from build123d import *

# Parameters (mm, degrees)
SKETCH_2_R           = 3
SKETCH_2_R_2         = 2.5
SKETCH_2_R_3         = 2.55
SKETCH_2_W           = 6
SKETCH_2_H           = 6
SKETCH_2_W_2         = 6.1
SKETCH_2_H_2         = 2
EXTRUDE_2_DEPTH      = 8.5
CHAMFER_3_SIZE       = 2.5
FILLET_1_R           = 3
CUT_EXTRUDE_1_DEPTH  = 1.2
SKETCH_4_R           = 0.85
CUT_EXTRUDE_2_DEPTH  = 5
CUT_EXTRUDE_3_DEPTH  = 1.2
SKETCH_6_R           = 0.85
CUT_EXTRUDE_4_DEPTH  = 5
FILLET_2_R           = 2
SKETCH_7_W           = 6.1
SKETCH_7_H           = 10
CUT_EXTRUDE_5_DEPTH  = 2
SKETCH_8_R           = 0.85
CUT_EXTRUDE_6_DEPTH  = 5
SKETCH_9_R           = 3.65
CUT_EXTRUDE_7_DEPTH  = 2.5
SKETCH_10_R          = 3.65
CUT_EXTRUDE_8_DEPTH  = 2.5
SKETCH_11_R          = 5
CUT_EXTRUDE_9_DEPTH  = 2.5
SKETCH_12_R          = 5
CUT_EXTRUDE_10_DEPTH = 2.5
CHAMFER_4_SIZE       = 0.5
CHAMFER_5_SIZE       = 0.3


with BuildPart() as part:
    # 草图2 → 凸台-拉伸2 (new body)
    with BuildSketch(Plane.XY):
        with BuildLine():
            Line((-10.9, 9.1), (25.9, 9.1))
            ThreePointArc((25.9, 9.1), (29.435533906, 10.564466094), (30.9, 14.1))
            Line((30.9, 14.1), (30.9, 29.1))
            ThreePointArc((30.9, 29.1), (32.364466094, 32.635533906), (35.9, 34.1))
            Line((35.9, 34.1), (44.1, 34.1))
            ThreePointArc((44.1, 34.1), (47.635533906, 32.635533906), (49.1, 29.1))
            Line((49.1, 29.1), (49.1, 9.1))
            Line((49.1, 9.1), (49.1, -45.9))
            ThreePointArc((49.1, -45.9), (47.635533906, -49.435533906), (44.1, -50.9))
            Line((44.1, -50.9), (-4.1, -50.9))
            ThreePointArc((-4.1, -50.9), (-7.635533906, -49.435533906), (-9.1, -45.9))
            Line((-9.1, -45.9), (-9.1, -14.1))
            ThreePointArc((-9.1, -14.1), (-10.564466094, -10.564466094), (-14.1, -9.1))
            Line((-14.1, -9.1), (-30.9, -9.1))
            ThreePointArc((-30.9, -9.1), (-34.435533906, -7.635533906), (-35.9, -4.1))
            Line((-35.9, -4.1), (-35.9, 4.1))
            ThreePointArc((-35.9, 4.1), (-34.435533906, 7.635533906), (-30.9, 9.1))
            Line((-30.9, 9.1), (-10.9, 9.1))
        make_face()
        Circle(SKETCH_2_R, mode=Mode.SUBTRACT)
        with Locations((40, 0)):
            Circle(SKETCH_2_R_2, mode=Mode.SUBTRACT)
        with Locations((0, -40)):
            Circle(SKETCH_2_R, mode=Mode.SUBTRACT)
        with Locations((40, -40)):
            Circle(SKETCH_2_R_3, mode=Mode.SUBTRACT)
        with Locations((40, 25)):
            Circle(SKETCH_2_R_3, mode=Mode.SUBTRACT)
        with Locations((-26.8, 0)):
            Circle(SKETCH_2_R_3, mode=Mode.SUBTRACT)
        with Locations((20, -20)):
            Rectangle(SKETCH_2_W, SKETCH_2_H, mode=Mode.SUBTRACT)
        with Locations((20, -40.9)):
            Rectangle(SKETCH_2_W_2, SKETCH_2_H_2, mode=Mode.SUBTRACT)
    extrude(amount=EXTRUDE_2_DEPTH)

    # 倒角3
    chamfer_3_edges = [part.edges().sort_by_distance(p)[0] for p in [
        (37.5, 0, 0),
        (37.45, -40, 8.5),
        (37.45, 25, 8.5),
        (-29.35, 0, 0),
    ]]
    chamfer(chamfer_3_edges, length=CHAMFER_3_SIZE)

    # 圆角1
    fillet_1_edges = [part.edges().sort_by_distance(p)[0] for p in [
        (20, -41.9, 0),
    ]]
    fillet(fillet_1_edges, radius=FILLET_1_R)

    # 草图3 → 切除-拉伸1 (cut)
    with BuildSketch(Plane.XY.offset(8.5)):
        with BuildLine():
            Line((15.9, -11.9), (24.1, -11.9))
            ThreePointArc((24.1, -11.9), (24.807106781, -12.192893219), (25.1, -12.9))
            Line((25.1, -12.9), (25.1, -27.1))
            ThreePointArc((25.1, -27.1), (24.807106781, -27.807106781), (24.1, -28.1))
            Line((24.1, -28.1), (15.9, -28.1))
            ThreePointArc((15.9, -28.1), (15.192893219, -27.807106781), (14.9, -27.1))
            Line((14.9, -27.1), (14.9, -12.9))
            ThreePointArc((14.9, -12.9), (15.192893219, -12.192893219), (15.9, -11.9))
        make_face()
    extrude(amount=-CUT_EXTRUDE_1_DEPTH, mode=Mode.SUBTRACT)

    # 草图4 → 切除-拉伸2 (cut)
    with BuildSketch(Plane.XY.offset(7.3)):
        with Locations((20, -14.3)):
            Circle(SKETCH_4_R)
        with Locations(Location((20, -25.7, 0), (0, 0, 180))):
            Circle(SKETCH_4_R)
    extrude(amount=-CUT_EXTRUDE_2_DEPTH, mode=Mode.SUBTRACT)

    # 草图5 → 切除-拉伸3 (cut)
    with BuildSketch(Plane(origin=(0, 0, 0), x_dir=(-1, 0, 0), z_dir=(0, 0, -1))):
        with BuildLine():
            Line((-27.1, -14.9), (-12.9, -14.9))
            ThreePointArc((-12.9, -14.9), (-12.192893219, -15.192893219), (-11.9, -15.9))
            Line((-11.9, -15.9), (-11.9, -24.1))
            ThreePointArc((-11.9, -24.1), (-12.192893219, -24.807106781), (-12.9, -25.1))
            Line((-12.9, -25.1), (-27.1, -25.1))
            ThreePointArc((-27.1, -25.1), (-27.807106781, -24.807106781), (-28.1, -24.1))
            Line((-28.1, -24.1), (-28.1, -15.9))
            ThreePointArc((-28.1, -15.9), (-27.807106781, -15.192893219), (-27.1, -14.9))
        make_face()
    extrude(amount=-CUT_EXTRUDE_3_DEPTH, mode=Mode.SUBTRACT)

    # 草图6 → 切除-拉伸4 (cut)
    with BuildSketch(Plane(origin=(0, 0, 1.2), x_dir=(-1, 0, 0), z_dir=(0, 0, -1))):
        with Locations((-25.7, -20)):
            Circle(SKETCH_6_R)
        with Locations(Location((-14.3, -20, 0), (0, 0, 180))):
            Circle(SKETCH_6_R)
    extrude(amount=-CUT_EXTRUDE_4_DEPTH, mode=Mode.SUBTRACT)

    # 圆角2
    fillet_2_edges = [part.edges().sort_by_distance(p)[0] for p in [
        (-35.9, 0, 8.5),
        (-34.435533906, -7.635533906, 8.5),
        (-2.5, 9.1, 0),
        (-22.5, -9.1, 8.5),
        (29.435533906, 10.564466094, 0),
        (30.9, 21.6, 0),
        (32.364466094, 32.635533906, 0),
        (40, 34.1, 0),
        (47.635533906, 32.635533906, 0),
        (49.1, -8.4, 0),
        (47.635533906, -49.435533906, 0),
        (-10.564466094, -10.564466094, 8.5),
        (20, -50.9, 0),
        (-7.635533906, -49.435533906, 0),
        (-9.1, -30, 0),
        (-10.564466094, -10.564466094, 0),
        (-22.5, -9.1, 0),
        (-34.435533906, -7.635533906, 0),
        (-35.9, 0, 0),
        (-9.1, -30, 8.5),
        (-34.435533906, 7.635533906, 0),
        (-7.635533906, -49.435533906, 8.5),
        (20, -50.9, 8.5),
        (47.635533906, -49.435533906, 8.5),
        (49.1, -8.4, 8.5),
        (-2.5, 9.1, 8.5),
        (47.635533906, 32.635533906, 8.5),
        (40, 34.1, 8.5),
        (32.364466094, 32.635533906, 8.5),
        (30.9, 21.6, 8.5),
        (29.435533906, 10.564466094, 8.5),
        (-34.435533906, 7.635533906, 8.5),
    ]]
    fillet(fillet_2_edges, radius=FILLET_2_R)

    # 草图7 → 切除-拉伸5 (cut)
    with BuildSketch(Plane(origin=(0, 0, 8.5), x_dir=(-1, 0, 0), z_dir=(0, 0, -1))):
        with Locations((-20, -41.9)):
            Rectangle(SKETCH_7_W, SKETCH_7_H)
    extrude(amount=CUT_EXTRUDE_5_DEPTH, mode=Mode.SUBTRACT)

    # 草图8 → 切除-拉伸6 (cut)
    with BuildSketch(Plane.XY.offset(6.5)):
        with Locations((20, -45.3)):
            Circle(SKETCH_8_R)
    extrude(amount=-CUT_EXTRUDE_6_DEPTH, mode=Mode.SUBTRACT)

    # 草图9 → 切除-拉伸7 (cut)
    with BuildSketch(Plane.XY.offset(8.5)):
        with Locations((0, -40)):
            Circle(SKETCH_9_R)
    extrude(amount=-CUT_EXTRUDE_7_DEPTH, mode=Mode.SUBTRACT)

    # 草图10 → 切除-拉伸8 (cut)
    with BuildSketch(Plane(origin=(0, 0, 0), x_dir=(-1, 0, 0), z_dir=(0, 0, -1))):
        Circle(SKETCH_10_R)
    extrude(amount=-CUT_EXTRUDE_8_DEPTH, mode=Mode.SUBTRACT)

    # 草图11 → 切除-拉伸9 (cut)
    with BuildSketch(Plane(origin=(0, 0, 0), x_dir=(-1, 0, 0), z_dir=(0, 0, -1))):
        with Locations((0, -40)):
            Circle(SKETCH_11_R)
    extrude(amount=-CUT_EXTRUDE_9_DEPTH, mode=Mode.SUBTRACT)

    # 草图12 → 切除-拉伸10 (cut)
    with BuildSketch(Plane.XY.offset(8.5)):
        Circle(SKETCH_12_R)
    extrude(amount=-CUT_EXTRUDE_10_DEPTH, mode=Mode.SUBTRACT)

    # 倒角4
    chamfer_4_edges = [part.edges().sort_by_distance(p)[0] for p in [
        (5, -40, 0),
        (-5, 0, 8.5),
    ]]
    chamfer(chamfer_4_edges, length=CHAMFER_4_SIZE)

    # 倒角5
    chamfer_5_edges = [part.edges().sort_by_distance(p)[0] for p in [
        (24.807106781, -27.807106781, 8.5),
        (25.1, -20, 8.5),
        (24.807106781, -12.192893219, 8.5),
        (20, -11.9, 8.5),
        (15.192893219, -12.192893219, 8.5),
        (14.9, -20, 8.5),
        (15.192893219, -27.807106781, 8.5),
        (20, -28.1, 8.5),
        (12.192893219, -15.192893219, 0),
        (20, -14.9, 0),
        (27.807106781, -15.192893219, 0),
        (28.1, -20, 0),
        (27.807106781, -24.807106781, 0),
        (20, -25.1, 0),
        (12.192893219, -24.807106781, 0),
        (11.9, -20, 0),
    ]]
    chamfer(chamfer_5_edges, length=CHAMFER_5_SIZE)


solid = part.part
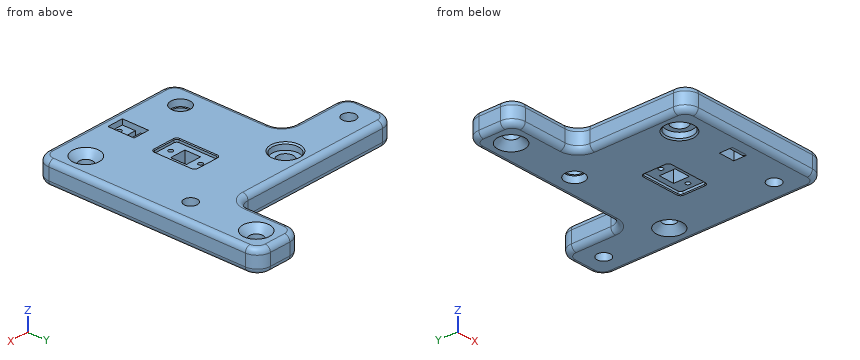
Source: CAD feature listing. Evaluate the final solid. Frame: model axes, mm. Round coordinates to 2 decimals unless told otherwise and drop trailing zeros. Write each loop counter-clockwise with the first axis right and the second up, starting at its lowest first coordinate (ties: lowest second). Pieces come first, ordered by that corner, then holes. Notation, with made-up numbers: M 19,23.25 L 71,23.25 A22 cw 71,52.25 Z; hole C 8.5,-16.75 d10. An arc over 180 degrees is marked long. One line per item, written item: value. Start each with the question number.
Item 1: Ray query, L1, parallel to Y at x = 0, z = 4.1; L2, parallel to Y at x = 40, z = 4.3; L3, parallel to X at y = -45.3, z = 4.95. Return the intervals inside material, ascending. Write a range as from..to.
Item 2: Section query C-C (x = 40). Return the cut outline in (y, z), plus the area to 3 significant figures.
Item 3: Section query B-B (y = 25). Return the cut outline in (x, z).
Item 4: Section query D-D (y = -29.5). Return the cut outline in (x, z), plus the area to 3 significant figures.
Item 5: Pin query (flat end, axial travel): pin 1 (6.5 mm diameter, centred on x = 40, y = 0, fed in from -Z); pin 2 (1 mm diameter, centred on x = 19.5, z = 5.5, fed in from +Y); pin 3 (2 mm diameter, centred on x = 2.5, z = 1.5, fed in from -Y); pin 4 (1 mm diameter, centred on x = 18.5, z = 0.5, fed in from +Y). Return the tip coordinate at first contact, or that it passes through.
Item 6: Section query A-A (x = -26.8). Return the cut outline in (y, z), plus the area to 3 significant figures.
Result set:
1. L1: y = -50.9..-43, -37..-3, 3..9.1
1. L2: y = -50.9..-42.55, -37.45..-2.5, 2.5..22.45, 27.55..34.1
1. L3: x = -9.1..19.15, 20.85..49.1
2. outline: M -50.9,2 A2 ccw -48.9,0 L -42.55,0 L -42.55,6 L -45.05,8.5 L -48.9,8.5 A2 ccw -50.9,6.5 Z; M -37.45,0 L -5,0 L -2.5,2.5 L -2.5,8.5 L -34.95,8.5 L -37.45,6 Z; M 2.5,2.5 L 5,0 L 22.45,0 L 22.45,6 L 19.95,8.5 L 2.5,8.5 Z; M 27.55,0 L 32.1,0 A2 ccw 34.1,2 L 34.1,6.5 A2 ccw 32.1,8.5 L 30.05,8.5 L 27.55,6 Z
2. area: 571 mm²
3. outline: M 30.9,2 A2 ccw 32.9,0 L 37.45,0 L 37.45,6 L 34.95,8.5 L 32.9,8.5 A2 ccw 30.9,6.5 Z; M 42.55,0 L 47.1,0 A2 ccw 49.1,2 L 49.1,6.5 A2 ccw 47.1,8.5 L 45.05,8.5 L 42.55,6 Z
4. outline: M -9.1,2 A2 ccw -7.1,0 L 47.1,0 A2 ccw 49.1,2 L 49.1,6.5 A2 ccw 47.1,8.5 L -7.1,8.5 A2 ccw -9.1,6.5 Z
4. area: 491 mm²
5. pin 1: stops at z = 1.75
5. pin 2: stops at y = 9.1
5. pin 3: stops at y = -50.9
5. pin 4: stops at y = 8.83
6. outline: M -9.1,2 A2 ccw -7.1,0 L -5.05,0 L -2.55,2.5 L -2.55,8.5 L -7.1,8.5 A2 ccw -9.1,6.5 Z; M 2.55,2.5 L 5.05,0 L 7.1,0 A2 ccw 9.1,2 L 9.1,6.5 A2 ccw 7.1,8.5 L 2.55,8.5 Z
6. area: 102 mm²
